from build123d import *

# Parameters (mm, degrees)
SKETCH1_W      = 10
SKETCH1_H      = 29.5
EXTRUDE1_DEPTH = 20
SKETCH2_R      = 2.45
EXTRUDE2_DEPTH = 30.5
SKETCH4_R      = 1.95
EXTRUDE3_DEPTH = 11
FILLET1_R      = 4


with BuildPart() as part:
    # Sketch1 → Extrude1 (new body)
    with BuildSketch(Plane.XY):
        with Locations((0.322019203, 1.164845717)):
            Rectangle(SKETCH1_W, SKETCH1_H)
    extrude(amount=EXTRUDE1_DEPTH)

    # Sketch2 → Extrude2 (cut, through all)
    with BuildSketch(Plane(origin=(0, 15.914845717, 0), x_dir=(-1, 0, 0), z_dir=(0, 1, 0))):
        with Locations((0, 16)):
            Circle(SKETCH2_R)
    extrude(amount=-EXTRUDE2_DEPTH, mode=Mode.SUBTRACT)

    # Sketch4 → Extrude3 (cut)
    with BuildSketch(Plane.XY):
        with Locations((0, 7.914845717)):
            Circle(SKETCH4_R)
        with Locations((0, -7.085154283)):
            Circle(SKETCH4_R)
    extrude(amount=EXTRUDE3_DEPTH, mode=Mode.SUBTRACT)

    # Fillet1
    fillet1_edges = [part.edges().sort_by_distance(p)[0] for p in [
        (5.322019203, 1.164845717, 20),
        (-4.677980797, 1.164845717, 20),
    ]]
    fillet(fillet1_edges, radius=FILLET1_R)


solid = part.part
Work out the finished part from the listing and answer in its coordinate system (mm). A direction names the side the tool comes from. Coordinates: 2 decimals unless noted, no trailing zeros. Loops run counter-clockwise (first coordinate to the right, second up) from the corner with the lowest first, then second, coordinate; pieces in that order, holes last. Notation, with made-up numbers: M 5.25,50.5 L 52.25,50.5 A20 cw 52.25,88.5 Z; hole C 5.25,23 d11. An arc over 180 degrees is marked long. Answer in a Markdown table with one row per item. Add a question column.
1. The mould has two halves that part along Y. Classify faces 1 (the cylindrical face through (-3.537, 1.371, 18.797)), 2 (the flat face through (0, 15.915, 10)), 3 (the cylindrical face through (-1.55, 6.73, 5.42)): pulls with the +Y half, pulls with the -Y half, needs draft (parallel to the pull), parting line crosses it, or undercut.
2. Find section C-C, the plane z = 3.75. Write down the section's boundary in (x, y).
3. Find section A-A, the plane y = 5.25. Write down the section's boundary in (x, z), then the cut area to 3 significant figures.
4. Find section B-B, the plane x = 0. Write down the section's boundary in (y, z), then the cut area to 3 significant figures.
5. Flat-ended cylindrical pins translate along their axes: P1, Ø3, axis at x = 0, y = -7.5, coming from the -Z side; P2, Ø1.5, axis at y = -6.5, z = 17, coming from the +X side. Find the tip coordinate at first contact, or state that the pin passes through.
6. Consider L1, parallel to Y at x = 0, z = 7.5; L2, parallel to Y at x = -1, z = 2; L3, parallel to Z at x = 0, y = 7. Determine where each line is inside the solid, lowest interval first.
7. Find section D-D, the plane x = 3.5. Write down the section's boundary in (y, z).
8. A tool of negligible diameter and unlimited length cuts with its end or side. For faces 4 (the flat face through (0, -7, 11)), 5 (the flat face through (0, 1, 20)), from which of +Z, -Z, +X, -X, +Y, -Y can it reach the whole face along a straight path? Write none if from no direction.
Reported:
| question | item | result |
|---|---|---|
| 1 | face 1 | needs draft |
| 1 | face 2 | pulls with the +Y half |
| 1 | face 3 | undercut |
| 2 | outline | M -4.68,-13.59 L 5.32,-13.59 L 5.32,15.91 L -4.68,15.91 Z; hole C 0,-7.09 d3.9; hole C 0,7.91 d3.9 |
| 3 | outline | M -4.68,0 L 5.32,0 L 5.32,16 A4 ccw 1.32,20 L -0.68,20 A4 ccw -4.68,16 Z; hole C 0,16 d4.9 |
| 3 | area | 174 mm^2 |
| 4 | outline | M -13.59,0 L -9.04,0 L -9.04,11 L -5.14,11 L -5.14,0 L 5.96,0 L 5.96,11 L 9.86,11 L 9.86,0 L 15.91,0 L 15.91,13.55 L -13.59,13.55 Z; M -13.59,18.45 L 15.91,18.45 L 15.91,20 L -13.59,20 Z |
| 4 | area | 360 mm^2 |
| 5 | P1 | stops at z = 11 |
| 5 | P2 | stops at x = 5.31 |
| 6 | L1 | y = -13.59 to -9.04, -5.14 to 5.96, 9.86 to 15.91 |
| 6 | L2 | y = -13.59 to -8.76, -5.41 to 6.24, 9.59 to 15.91 |
| 6 | L3 | z = 11 to 13.55, 18.45 to 20 |
| 7 | outline | M -13.59,0 L 15.91,0 L 15.91,19.36 L -13.59,19.36 Z |
| 8 | face 4 | -Z |
| 8 | face 5 | +Z, +X, -X, +Y, -Y |
